from build123d import *

# Parameters (mm, degrees)
F0_W     = 203.2
F0_H     = 127
F1_DEPTH = 127
F3_DEPTH = 76.2
F4_SIZE2 = 101.6
F4_SIZE  = 76.2
F5_R     = 5.08
F6_R     = 15.24
F7_DEPTH = 50.801
F8_R     = 21.8504369972
F9_DEPTH = 127.001


with BuildPart() as f1:
    # F0 (on Front) → F1 (new body)
    with BuildSketch(Plane.XZ):
        with Locations((3.2226219773, -13.3488786947)):
            Rectangle(F0_W, F0_H)
    extrude(amount=F1_DEPTH)

    # F2 (on face) → F3 (cut)
    with BuildSketch(Plane.XZ.offset(127)):
        Polygon((-34.8773780227, -13.3488786947), (-34.8773780227, -76.8488786947), (104.8226219773, -76.8488786947), (104.8226219773, 50.1511213053), (3.2226219773, 50.1511213053), (3.2226219773, -13.3488786947), align=None)
    extrude(amount=-F3_DEPTH, mode=Mode.SUBTRACT)

    # F4
    f4_edges = [f1.edges().sort_by_distance(p)[0] for p in [
        (104.822622, -25.4, 50.151121),
    ]]
    f4_side = f1.faces().sort_by_distance((-18.548807, -52.614286, 50.151121))[0]
    chamfer(f4_edges, length=F4_SIZE, length2=F4_SIZE2, reference=f4_side)

    # F5
    f5_edges = [f1.edges().sort_by_distance(p)[0] for p in [
        (3.222622, -88.9, 50.151121),
        (-47.577378, -127, 50.151121),
        (-34.877378, 0, 50.151121),
        (28.622622, -25.4, 50.151121),
        (-98.377378, -63.5, 50.151121),
        (15.922622, -50.8, 50.151121),
        (3.222622, -88.9, -13.348879),
        (-34.877378, -88.9, -13.348879),
        (-15.827378, -127, -13.348879),
        (-15.827378, -50.8, -13.348879),
        (3.222622, -127, 18.401121),
        (3.222622, -50.8, 18.401121),
        (-34.877378, -88.9, -76.848879),
        (-34.877378, -127, -45.098879),
        (-34.877378, -50.8, -45.098879),
        (104.822622, 0, -64.148879),
        (104.822622, -25.4, -51.448879),
        (104.822622, -25.4, -76.848879),
        (104.822622, -50.8, -64.148879),
        (3.222622, 0, -76.848879),
        (34.972622, -50.8, -76.848879),
        (-66.627378, -127, -76.848879),
        (-98.377378, -63.5, -76.848879),
        (-98.377378, 0, -13.348879),
        (-98.377378, -127, -13.348879),
    ]]
    fillet(f5_edges, radius=F5_R)

    # F6 (on face) → F7 (cut, through all)
    with BuildSketch(Plane.XZ.offset(50.8)):
        with Locations((21.0026219773, -31.1288786947)):
            Circle(F6_R)
    extrude(amount=-F7_DEPTH, mode=Mode.SUBTRACT)

    # F8 (on face) → F9 (cut, through all)
    with BuildSketch(Plane.XY.offset(50.1511213053)):
        with Locations((-66.7120441794, -63.0343332887)):
            Circle(F8_R)
    extrude(amount=-F9_DEPTH, mode=Mode.SUBTRACT)


solid = f1.part
Verification items for the finished model (mm, model axes). A direction names the side the tool comes from. Give positions to 0.01 mm unless a question says otherwise; leave off trailing zeros. Loops run counter-clockwise (first coordinate to the right, second up) from the corner with the lowest first, then second, coordinate; pieces in that order, holes last. Notation, with made-up numbers: (64, -15) - (86, -15) arc R24 ccw to (86, -3) - close; hole circle Ø5 at (-15, 57.25). An arc over 180 degrees is marked (long way). Write item = value, one per line. Start each with the question number.
Q1. Tool access check on faces 4 (the face through (-16.02, -125.55, -11.82)), 5 (the face through (3.223, -89, 19)), 6 (the face through (-46.937, -125.472, 48.703)). Record the directions out of +Z, -Z, +X, -X, +Y, -Y that give a thin tool (end or side, any length) a straight path to the whole face; none if there is none.
Q2. Cross-section at C-C, the plane y = -95. Enter the section's corners in (x, z).
Q3. Cross-section at A-A, the plane z = -25. Enter the section's corners in (x, y).
Q4. Cross-section at D-D, the plane z = -67. Enter the section's corners in (x, y).
Q5. Depth check by flat-ended pin: P1, Ø3, axis at y = -78, z = -7.5, coming from the +X side; P2, Ø1.5, axis at x = 32, z = -45, coming from the -Y side; P3, Ø18.5, axis at x = 21, z = -31.13, coming from the +Y side. Enter the tip coordinate at first touch or a pass-through.
Q6. Cross-section at B-B, the plane x = -9. Enter the section's corners in (y, z).
Q7. Thickness scan on line 1 (X direction, y = -62, z = 33); line 2 (Y direction, x = -66.5, z = 28); line 3 (X direction, y = -106, z = -45.5). Record the ranges inside material, lowest first.
Q8. Mould release check, pull along Z, two halves, no side actions. Record for faces 1 (the face through (35.54, -25.76, -26.55)), 2 (the face through (17.518, -49.272, 48.703)), 3 (the face through (103.295, -49.351, -61.043)): released by +Z, released by -Z, zero draft, split by the parting line, or undercut.
Answer key:
q1.face_4 = -Z, +X, -Y
q1.face_5 = +Z, -Z, +X, -Y
q1.face_6 = +Z, +X, -X, -Y
q2.outline = (-98.38, -71.77) arc R5.08 ccw to (-93.3, -76.85) - (-39.96, -76.85) arc R5.08 ccw to (-34.88, -71.77) - (-34.88, -18.43) arc R5.08 cw to (-29.8, -13.35) - (-1.86, -13.35) arc R5.08 ccw to (3.22, -8.27) - (3.22, 45.07) arc R5.08 ccw to (-1.86, 50.15) - (-93.3, 50.15) arc R5.08 ccw to (-98.38, 45.07) - close
q3.outline = (-98.38, -121.92) arc R5.08 ccw to (-93.3, -127) - (-39.96, -127) arc R5.08 ccw to (-34.88, -121.92) - (-34.88, -55.88) arc R5.08 cw to (-29.8, -50.8) - (7.05, -50.8) - (7.05, 0) - (-93.3, 0) arc R5.08 ccw to (-98.38, -5.08) - close; (34.96, -50.8) - (84.99, -50.8) - (84.99, 0) - (34.96, 0) - close; hole circle Ø43.7 at (-66.71, -63.03)
q4.outline = (-98.38, -121.92) arc R5.08 ccw to (-93.3, -127) - (-39.96, -127) arc R5.08 ccw to (-34.88, -121.92) - (-34.88, -55.88) arc R5.08 cw to (-29.8, -50.8) - (99.74, -50.8) arc R5.08 ccw to (104.82, -45.72) - (104.82, -5.08) arc R5.08 ccw to (99.74, 0) - (-93.3, 0) arc R5.08 ccw to (-98.38, -5.08) - close; hole circle Ø43.7 at (-66.71, -63.03)
q5.P1 = 3.22
q5.P2 = -50.8
q5.P3 = through
q6.outline = (-127, -8.27) arc R5.08 ccw to (-121.92, -13.35) - (-55.88, -13.35) arc R5.08 cw to (-50.8, -18.43) - (-50.8, -71.77) arc R5.08 ccw to (-45.72, -76.85) - (-5.08, -76.85) arc R5.08 ccw to (0, -71.77) - (0, 45.07) arc R5.08 ccw to (-5.08, 50.15) - (-121.92, 50.15) arc R5.08 ccw to (-127, 45.07) - close
q7.line_1 = -98.38 to -88.54, -44.89 to 3.22
q7.line_2 = -127 to -84.88, -41.18 to 0
q7.line_3 = -98.38 to -34.88
q8.face_1 = undercut
q8.face_2 = released by +Z
q8.face_3 = zero draft
